Model file for the job. Use its own axes, mm. Face numbers are marked on the shaded views. A direction names the side the tool comes from. Give positions to 0.01 mm unless a question says otherwise; leave off trailing zeros. Write each loop counter-clockwise with the first axis right and the second up, starting at its lowest first coordinate (ties: lowest second). Pieces come first, ordered by that corner, then holes. Notation, with made-up numbers: (50, 85) - (71, 85) arc R26 ccw to (71, 101) - close; hole circle Ø7 at (-31.5, 54). An arc over 180 degrees is marked (long way). Use a Markdown table: item, result. Add a question column.
```python
from build123d import *

# Parameters (mm, degrees)
SKETCH1_R                = 24.193
SKETCH1_R_2              = 20.193
BOSS_EXTRUDE1_DEPTH      = 24
CUT_EXTRUDE1_DEPTH       = 24
BOSS_EXTRUDE2_DEPTH      = 24
SKETCH4_R                = 4
CUT_EXTRUDE2_DEPTH       = 24
SKETCH5_R                = 3
BOSS_EXTRUDE3_DEPTH      = 24
CUT_EXTRUDE3_DEPTH       = 37
SKETCH7_W                = 4.5
SKETCH7_H                = 37.5
CUT_EXTRUDE4_DEPTH       = 0.5
SKETCH8_W                = 23.824241379
SKETCH8_H                = 4.5
BOSS_EXTRUDE4_DEPTH      = 6.5
BOSS_EXTRUDE4_DEPTH_BACK = 1


with BuildPart() as part:
    # Sketch1 → Boss-Extrude1 (new body)
    with BuildSketch(Plane.XY):
        Circle(SKETCH1_R)
        Circle(SKETCH1_R_2, mode=Mode.SUBTRACT)
    extrude(amount=BOSS_EXTRUDE1_DEPTH)

    # Sketch2 → Cut-Extrude1 (cut)
    with BuildSketch(Plane.XY.offset(24)):
        Polygon((0, -24.193), (-5.8341998, -24.895299835), (-12.0965, -20.951752594), (0, 0), align=None)
    extrude(amount=-CUT_EXTRUDE1_DEPTH, mode=Mode.SUBTRACT)

    # Sketch3 → Boss-Extrude2 (add)
    with BuildSketch(Plane.XY.offset(24)):
        with BuildLine():
            Line((-15.990029306, -35.482601784), (-12.0965, -20.951752594))
            ThreePointArc((-12.0965, -20.951752594), (-14.346719144, -19.480064138), (-16.419734671, -17.767767512))
            Line((-16.419734671, -17.767767512), (-20.819658437, -34.188506559))
            Line((-20.819658437, -34.188506559), (-15.990029306, -35.482601784))
        make_face()
        with BuildLine():
            ThreePointArc((5.336023592, -23.597205369), (2.684591171, -24.043589982), (0, -24.193))
            Line((0, -24.193), (-3.893529306, -38.72384919))
            Line((-3.893529306, -38.72384919), (0.936099826, -40.017944416))
            Line((0.936099826, -40.017944416), (5.336023592, -23.597205369))
        make_face()
    extrude(amount=-BOSS_EXTRUDE2_DEPTH)

    # Sketch4 → Cut-Extrude2 (cut)
    with BuildSketch(Plane(origin=(-10.877879131, 2.914718929, 0), x_dir=(0, 0, 1), z_dir=(-0.965925826, 0.258819045, 0))):
        with Locations((12, -30.412085563)):
            Circle(SKETCH4_R)
    extrude(amount=-CUT_EXTRUDE2_DEPTH, mode=Mode.SUBTRACT)

    # Sketch5 → Boss-Extrude3 (add)
    with BuildSketch(Plane.XY.offset(24)):
        Polygon((16.953408399, 17.259292937), (31.579228629, 71.843597138), (8.640561787, 78.258704162), (-6.052435886, 23.423690334), align=None)
        with Locations((23.835868108, 68.298098762)):
            Circle(SKETCH5_R, mode=Mode.SUBTRACT)
        with Locations((13.421299193, 71.210673179)):
            Circle(SKETCH5_R, mode=Mode.SUBTRACT)
    extrude(amount=-BOSS_EXTRUDE3_DEPTH)

    # Sketch6 → Cut-Extrude3 (cut)
    with BuildSketch(Plane(origin=(20.925291279, 74.82311416, 0), x_dir=(0.963048124, -0.269329374, 0), z_dir=(0.269329374, 0.963048124, 0))):
        Polygon((-0.846682582, -9.75), (-12.756090991, -9.75), (-12.756090991, -14.25), (-0.846682582, -14.25), (11.062725828, -14.25), (11.062725828, -9.75), align=None)
    extrude(amount=-CUT_EXTRUDE3_DEPTH, mode=Mode.SUBTRACT)

    # Sketch7 → Cut-Extrude4 (cut)
    with BuildSketch(Plane(origin=(11.502922142, -3.082198699, 0), x_dir=(0, 0, -1), z_dir=(0.965925826, -0.258819045, 0))):
        with Locations((-12, 58.818891727)):
            Rectangle(SKETCH7_W, SKETCH7_H)
    extrude(amount=-CUT_EXTRUDE4_DEPTH, mode=Mode.SUBTRACT)

    # Sketch8 → Boss-Extrude4 (add, two sides)
    with BuildSketch(Plane(origin=(10.960104439, 39.190333589, 0), x_dir=(0.963048124, -0.269329374, 0), z_dir=(0.269329374, 0.963048124, 0))) as boss_extrude4_sk:
        with Locations((-0.44075727, -12)):
            Rectangle(SKETCH8_W, SKETCH8_H)
    extrude(amount=BOSS_EXTRUDE4_DEPTH)
    extrude(boss_extrude4_sk.sketch, amount=-BOSS_EXTRUDE4_DEPTH_BACK)


solid = part.part
```
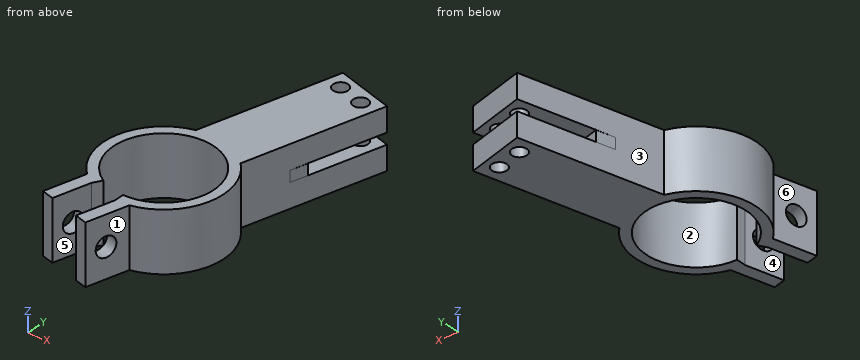
(1) Band-saw the part on A-A (y = 0). Write the cut outline in (x, z).
(2) Two-plate mould, pull along Y, no slides. Class the marked faces 1, 2 and 3: +Y half, -Y half, draft (parallel to the pull), parting line (faces both ways), or undercut.
(3) Band-saw the part on C-C (y = 47). Write the cut outline in (x, z).
(4) Probe probe 1 along X at (y, z) = (71, 5.5); probe 2 along Y at (x, z) = (15.5, 5.5); probe 3 along X at (y, z) = (0, 11.5). List the from-to ranges inside material, lowest first. Write a range as [from, to].
(5) Band-saw the part on B-B (z = 21.75). Write the cut outline in (x, y), then the cut area to 3 significant figures.
(6) Which spindle directions (+Z, -Z, +X, -X, +Y, -Y) get a long thin tool onto all of the face, cutting with end or side? Do the marked faces 4, 5 and 6. Say none if no direction does.
(7) Flat gauge pins, fed straight in: pin 1 (1.5 mm diameter, centred on x = 17, z = 11.5, fed in from -Y); pin 2 (3 mm diameter, centred on y = -22.5, z = 16.5, fed in from -X); pin 3 (12 mm diameter, centred on x = 17, z = 12, fed in from -Y); pin 4 (3.5 mm diameter, centred on x = 23.84, y = 68.3, fed in from +Z). Where does each tip first touch, or does it go through?
(8) Band-saw the part on D-D (x = -7.5). Write the cut outline in (y, z), then the cut area to 3 significant figures.
Model answer:
| question | item | result |
|---|---|---|
| 1 | outline | (-24.19, 0) - (-20.19, 0) - (-20.19, 24) - (-24.19, 24) - close; (20.19, 0) - (24.19, 0) - (24.19, 24) - (20.19, 24) - close |
| 2 | face 1 | -Y half |
| 2 | face 2 | undercut |
| 2 | face 3 | +Y half |
| 3 | outline | (0.26, 0) - (24.92, 0) - (24.92, 9.75) - (7.17, 9.75) - (7.17, 14.25) - (24.92, 14.25) - (24.92, 24) - (0.26, 24) - (0.26, 14.25) - (0.32, 14.25) - (0.32, 9.75) - (0.26, 9.75) - close |
| 4 | probe 1 | x = [6.7, 10.43], [16.41, 22.53], [25.14, 31.35] |
| 4 | probe 2 | y = [-18.58, -12.94], [12.94, 69.05], [73.37, 76.34] |
| 4 | probe 3 | x = [-24.19, -20.19], [20.19, 24.19] |
| 5 | outline | (-20.82, -34.19) - (-15.99, -35.48) - (-12.1, -20.95) - (-10.1, -17.49) arc R20.19 cw (long way) to (0, -20.19) - (0, -24.19) - (-3.89, -38.72) - (0.94, -40.02) - (5.34, -23.6) arc R24.19 ccw to (16.95, 17.26) - (31.58, 71.84) - (8.64, 78.26) - (-6.05, 23.42) arc R24.19 ccw to (-16.42, -17.77) - close; hole circle Ø6 at (13.42, 71.21); hole circle Ø6 at (23.84, 68.3) |
| 5 | area | 1,910 mm^2 |
| 6 | face 4 | +Z, -Z |
| 6 | face 5 | +Z, -Z, -Y |
| 6 | face 6 | +Z, -Z, -X |
| 7 | pin 1 | stops at y = -17.92 |
| 7 | pin 2 | stops at x = -18.09 |
| 7 | pin 3 | stops at y = -21.55 |
| 7 | pin 4 | passes through |
| 8 | outline | (18.75, 0) - (23, 0) - (23, 24) - (18.75, 24) - close |
| 8 | area | 102 mm^2 |
